Geometry check sheet. Reference: the model listing, model coordinates, mm. A direction names the side the tool comes from. Coordinates: 2 decimals unless noted, no trailing zeros. Write each loop counter-clockwise with the first axis right and the second up, starting at its lowest first coordinate (ties: lowest second). Pieces come first, ordered by that corner, then holes. Notation, with made-up numbers: (2.25, 51) -> (34.25, 51) arc R25 cw to (34.25, 81) -> close; hole circle Ø5 at (72, 88). An arc over 180 degrees is marked (long way). One line per question, with ' | ' between items.
from build123d import *

# Parameters (mm, degrees)
F1_DEPTH = 3.175
F2_R     = 3.9751
F2_R_2   = 3.175
F3_DEPTH = 3.176


with BuildPart() as f1:
    # F0 (on Front) → F1 (new body)
    with BuildSketch(Plane.XZ):
        with BuildLine():
            ThreePointArc((-1.133856, -15.7071281452), (10.7271510596, -11.5294290467), (15.748, 0))
            ThreePointArc((15.748, 0), (10.7271378512, 11.529441336), (-1.1338919889, 15.7071255473))
            ThreePointArc((-1.1338919889, 15.7071255473), (-11.529441336, 10.7271378512), (-15.748, 0))
            ThreePointArc((-15.748, 0), (-11.5294290467, -10.7271510596), (-1.133856, -15.7071281452))
        make_face()
        with BuildLine():
            ThreePointArc((-15.748, 0), (-11.529441336, 10.7271378512), (-1.1338919889, 15.7071255473))
            Line((-1.1338919889, 15.7071255473), (-45.34766523, 12.5153484696))
            ThreePointArc((-45.34766523, 12.5153484696), (-51.0602172111, 14.4088260903), (-53.7668572171, 19.7840105071))
            Line((-53.7668572171, 19.7840105071), (-55.6477540074, 45.0349007362))
            ThreePointArc((-55.6477540074, 45.0349007362), (-55.6314403813, 44.7426525705), (-55.626, 44.45))
            ThreePointArc((-55.626, 44.45), (-57.9322412049, 38.8822412049), (-63.5, 36.576))
            ThreePointArc((-63.5, 36.576), (-69.270857002, 39.0930339311), (-71.352244132, 45.0349257143))
            Line((-71.352244132, 45.0349257143), (-74.6451207035, 0.8302171429))
            ThreePointArc((-74.6451207035, 0.8302171429), (-63.0846043948, 11.1682775078), (-52.324, 0))
            ThreePointArc((-52.324, 0), (-55.887183119, -8.1821754525), (-64.304672, -11.1469941676))
            Line((-64.304672, -11.1469941676), (-1.133856, -15.7071281452))
            ThreePointArc((-1.133856, -15.7071281452), (-11.5294290467, -10.7271510596), (-15.748, 0))
        make_face()
        with BuildLine():
            ThreePointArc((-74.6451207035, 0.8302171429), (-71.9594789501, -7.3034369917), (-64.304672, -11.1469941676))
            ThreePointArc((-64.304672, -11.1469941676), (-55.887183119, -8.1821754525), (-52.324, 0))
            ThreePointArc((-52.324, 0), (-63.0846043948, 11.1682775078), (-74.6451207035, 0.8302171429))
        make_face()
        with BuildLine():
            ThreePointArc((-55.626, 44.45), (-55.6314403813, 44.7426525705), (-55.6477540074, 45.0349007362))
            ThreePointArc((-55.6477540074, 45.0349007362), (-63.4999874763, 52.324), (-71.352244132, 45.0349257143))
            ThreePointArc((-71.352244132, 45.0349257143), (-69.270857002, 39.0930339311), (-63.5, 36.576))
            ThreePointArc((-63.5, 36.576), (-57.9322412049, 38.8822412049), (-55.626, 44.45))
        make_face()
    extrude(amount=F1_DEPTH)

    # F2 (on face) → F3 (cut, through all)
    with BuildSketch(Plane.XZ.offset(3.175)):
        Circle(F2_R)
        with Locations((-63.5, 0)):
            Circle(F2_R_2)
        with Locations((-42.8498, 0)):
            Circle(F2_R_2)
        with Locations((-63.5, 44.45)):
            Circle(F2_R_2)
    extrude(amount=-F3_DEPTH, mode=Mode.SUBTRACT)


solid = f1.part
1. Cross-section at C-C on z = -2. Record the boundary of the cut face in (x, y) (3 decimals), and give its area (3 significant figures).
Worked answers:
outline: (-74.496, -3.175) -> (-65.966, -3.175) -> (-65.966, 0) -> (-74.496, 0) -> close; (-61.034, -3.175) -> (-45.316, -3.175) -> (-45.316, 0) -> (-61.034, 0) -> close; (-40.384, -3.175) -> (-3.435, -3.175) -> (-3.435, 0) -> (-40.384, 0) -> close; (3.435, -3.175) -> (15.62, -3.175) -> (15.62, 0) -> (3.435, 0) -> close | area: 233 mm²
2. Cross-section at A-A on y = -2.3. Record the boundary of the cut face in (x, z) (3 decimals), and give its area (3 significant figures).
Worked answers:
outline: (-74.645, 0.83) arc R11.176 ccw to (-64.305, -11.147) -> (-1.134, -15.707) arc R15.748 ccw (long way) to (-1.134, 15.707) -> (-45.348, 12.515) arc R7.874 cw to (-53.767, 19.784) -> (-55.648, 45.035) arc R7.874 ccw to (-71.352, 45.035) -> close; hole circle Ø6.35 at (-63.5, 0); hole circle Ø6.35 at (-63.5, 44.45); hole circle Ø6.35 at (-42.85, 0); hole circle Ø7.95 at (0, 0) | area: 2,890 mm²
3. Mould release check, pull along X, two halves, no side actions. Record for faces 1 (the face through (-60.47, -1.61, 0.95)), 2 (the face through (-40, 0, 11)), 3 (the face through (-54.694, -1.565, 32.233)): released by +X, released by -X, zero draft, split by the parting line, or undercut.
Worked answers:
face 1: undercut | face 2: zero draft | face 3: released by +X
4. Tool access check on faces 4 (the face through (-39.82, -1.61, 0.95)), 5 (the face through (-50.99, -1.57, 14.35)). Record the directions out of +Z, -Z, +X, -X, +Y, -Y that give a thin tool (end or side, any length) a straight path to the whole face; none if there is none.
Worked answers:
face 4: +Y, -Y | face 5: +Z, +Y, -Y
5. Material ranges on line 1 (Z direction, x = 0, y = -2.35); line 2 (Z direction, x = -1.5, y = -2.95); line 3 (Z direction, x = -30.5, y = -0.6), recorded low to high. Write a range as from..to.
Worked answers:
line 1: -15.75..-3.98, 3.98..15.75 | line 2: -15.68..-3.68, 3.68..15.68 | line 3: -13.59..13.59
6. Cross-section at B-B on x = 0. Record the boundary of the cut face in (y, z) (3 decimals).
Worked answers:
outline: (-3.175, -15.748) -> (0, -15.748) -> (0, -3.975) -> (-3.175, -3.975) -> close; (-3.175, 3.975) -> (0, 3.975) -> (0, 15.748) -> (-3.175, 15.748) -> close
7. Cross-section at D-D on z = 32. Record the boundary of the cut face in (x, y) (3 decimals), and give its area (3 significant figures).
Worked answers:
outline: (-72.323, -3.175) -> (-54.677, -3.175) -> (-54.677, 0) -> (-72.323, 0) -> close | area: 56.0 mm²
